Work out the finished part from the listing and answer in its coordinate system (mm). A direction names the side the tool comes from. Round coordinates to 2 decimals unless told otherwise and drop trailing zeros. Order: outer loops, then holes, each group sorted by start corner. A loop starts at its lowest first (then second) coordinate and runs counter-clockwise, first axis right, second up.
from build123d import *

# Parameters (mm, degrees)
BOSS_EXTRUDE1_DEPTH = 31
BOSS_EXTRUDE2_START = 22
BOSS_EXTRUDE2_DEPTH = 9
BOSS_EXTRUDE3_START = -22
BOSS_EXTRUDE3_DEPTH = 9
CUT_EXTRUDE1_DEPTH  = 39
CUT_EXTRUDE2_DEPTH  = 39


with BuildPart() as part:
    # Sketch1 → Boss-Extrude1 (new, symmetric)
    with BuildSketch(Plane.XY):
        Polygon((20, 16), (50, 16), (50, 0), (34, 0), (34, 6), (16, 6), (16, 0), (0, 0), (0, 42), (20, 42), align=None)
    extrude(amount=BOSS_EXTRUDE1_DEPTH, both=True)

    # Sketch1_3 → Boss-Extrude2 (add)
    with BuildSketch(Plane.XY.offset(BOSS_EXTRUDE2_START)):
        Polygon((20, 42), (20, 16), (50, 16), align=None)
    extrude(amount=BOSS_EXTRUDE2_DEPTH)

    # Sketch1_5 → Boss-Extrude3 (add)
    with BuildSketch(Plane.XY.offset(BOSS_EXTRUDE3_START)):
        Polygon((20, 42), (20, 16), (50, 16), align=None)
    extrude(amount=-BOSS_EXTRUDE3_DEPTH)

    # Sketch3 → Cut-Extrude1 (cut)
    with BuildSketch(Plane(origin=(20, 0, 0), x_dir=(0, 0, -1), z_dir=(1, 0, 0))):
        Polygon((-15, 42), (0, 27), (15, 42), align=None)
    extrude(amount=-CUT_EXTRUDE1_DEPTH, mode=Mode.SUBTRACT)

    # Sketch4 → Cut-Extrude2 (cut)
    with BuildSketch(Plane(origin=(0, 16, 0), x_dir=(1, 0, 0), z_dir=(0, 1, 0))):
        Polygon((50, 9), (41, 0), (50, -9), align=None)
    extrude(amount=-CUT_EXTRUDE2_DEPTH, mode=Mode.SUBTRACT)


solid = part.part
Item 1: Find section B-B (y = 14). Write down the section's boundary in (x, z).
Item 2: Given pin 1 (15 mm diameter, centred on x = 35.5, z = 9, fed in from +Y); pin 2 (3 mm diameter, centred on y = 8, z = 22.5, fed in from -X), each flat-ended and moving along its own axis, determine where each tip first touches the part or whether it passes through.
Item 3: Find section A-A (x = 42.5). Write down the section's boundary in (y, z), plus the area to 3 significant figures.
Item 4: A tool of negligible diameter and unlimited length cuts with its end or side. For faces 1 (the face through (10, 35, 8)), 2 (the face through (25, 6, 0)), 3 (the face through (40, 0, 0)), 4 (the face through (20, 26, 0)), 5 (the face through (46, 8, -5)), from which of +Z, -Z, +X, -X, +Y, -Y can it reach the whole face along a straight path? Write none if from no direction.
Item 5: Find section C-C (z = 24). Write down the section's boundary in (x, y), plus the area to 3 significant figures.
Item 6: For a pull along X with two mould halves and no side action, classify faces 6 (the face through (10, 34, -7)), 7 (the face through (0, 21, 0)), 8 (the face through (34, 3, 0)) as released by +X, released by -X, zero draft, split by the parting line, or undercut.
Item 7: Find the intervals of material crossed by line 1 along Z through (x, y) = (32, 21.5); line 2 along X through (y, z) = (5, -25); line 3 along X through (y, z) = (39.5, 19), in increasing order.
Item 8: Find section D-D (x = 13). Write down the section's boundary in (y, z).
Model answer:
1. outline: (0, -31) - (50, -31) - (50, -9) - (41, 0) - (50, 9) - (50, 31) - (0, 31) - close
2. pin 1: stops at y = 16
2. pin 2: stops at x = 0
3. outline: (0, -31) - (22.5, -31) - (22.5, -22) - (16, -22) - (16, -1.5) - (0, -1.5) - close; (0, 1.5) - (16, 1.5) - (16, 22) - (22.5, 22) - (22.5, 31) - (0, 31) - close
3. area: 1,060 mm2
4. face 1: +X, -X, +Y
4. face 2: +Z, -Z, -Y
4. face 3: +Z, -Z, +X, -X, -Y
4. face 4: +X, +Y
4. face 5: +X, +Y, -Y
5. outline: (0, 0) - (16, 0) - (16, 6) - (34, 6) - (34, 0) - (50, 0) - (50, 16) - (20, 42) - (0, 42) - close
5. area: 1,600 mm2
6. face 6: zero draft
6. face 7: released by -X
6. face 8: undercut
7. line 1: z = -31 to -22, 22 to 31
7. line 2: x = 0 to 16, 34 to 50
7. line 3: x = 0 to 20
8. outline: (0, -31) - (42, -31) - (42, -15) - (27, 0) - (42, 15) - (42, 31) - (0, 31) - close
